CAD build for the part. Positions are in the model's coordinates, mm. A direction names the side the tool comes from. Round coordinates to 2 decimals unless told otherwise and drop trailing zeros. Order: outer loops, then holes, each group sorted by start corner. A loop starts at its lowest first (then second) coordinate and runs counter-clockwise, first axis right, second up. Notation, with made-up numbers: M -39,78 L -24,78 A30 cw -24,105 Z; hole C 23,-8.5 d9. An arc over 180 degrees is marked long. Answer as CSV lines item,"result". Start each with the question number.
```python
from build123d import *

# Parameters (mm, degrees)
BOSS_EXTRUDE2_DEPTH      = 25.4
CUT_EXTRUDE2_START       = 50.900485433
CUT_EXTRUDE2_OUTLINE_W   = 50.8
CUT_EXTRUDE2_OUTLINE_H   = 25.4
CUT_EXTRUDE2_OUTLINE_W_2 = 44.45
CUT_EXTRUDE2_OUTLINE_H_2 = 19.05
CUT_EXTRUDE2_DEPTH       = 80


# Read off the part's stored shape, not the designer's step: Cut-Extrude2
with BuildPart() as part:
    # Sketch2 → Boss-Extrude2 (new body)
    with BuildSketch(Plane.XY):
        with BuildLine():
            Line((-25.4, 130.900485433), (25.4, 130.900485433))
            Line((25.4, 130.900485433), (25.4, 30.900485433))
            ThreePointArc((25.4, 30.900485433), (0, -40), (-25.4, 30.900485433))
            Line((-25.4, 30.900485433), (-25.4, 130.900485433))
        make_face()
        Polygon((-16.541112452, 22.766888123), (-10.26013758, 21.772079433), (-4.496681536, 23.64473982), (0, 28.141421356), (4.496681536, 23.64473982), (10.26013758, 21.772079433), (16.541112452, 22.766888123), (17.535921141, 16.485913251), (21.09793287, 11.583224708), (26.764082159, 8.696177445), (23.877034895, 3.030028156), (23.877034895, -3.030028156), (26.764082159, -8.696177445), (21.09793287, -11.583224708), (17.535921141, -16.485913251), (16.541112452, -22.766888123), (10.26013758, -21.772079433), (4.496681536, -23.64473982), (0, -28.141421356), (-4.496681536, -23.64473982), (-10.26013758, -21.772079433), (-16.541112452, -22.766888123), (-17.535921141, -16.485913251), (-21.09793287, -11.583224708), (-26.764082159, -8.696177445), (-23.877034895, -3.030028156), (-23.877034895, 3.030028156), (-26.764082159, 8.696177445), (-21.09793287, 11.583224708), (-17.535921141, 16.485913251), align=None, mode=Mode.SUBTRACT)
    extrude(amount=BOSS_EXTRUDE2_DEPTH)

    # Cut-Extrude2 outline → Cut-Extrude2 (cut)
    with BuildSketch(Plane(origin=(0, 0, 0), x_dir=(1, 0, 0), z_dir=(0, 1, 0)).offset(CUT_EXTRUDE2_START)):
        with Locations((0, -12.7)):
            Rectangle(CUT_EXTRUDE2_OUTLINE_W, CUT_EXTRUDE2_OUTLINE_H)
        with Locations((0, -12.7)):
            Rectangle(CUT_EXTRUDE2_OUTLINE_W_2, CUT_EXTRUDE2_OUTLINE_H_2, mode=Mode.SUBTRACT)
    extrude(amount=CUT_EXTRUDE2_DEPTH, mode=Mode.SUBTRACT)


solid = part.part
```
Q1. Mould opens along X. For faces 4 (the cylindrical face through (1.374, -39.976, 12.522)), 5 (the flat face through (-2.22, -25.92, 12.52)), 6 (the flat face through (0, 90, 22.225)), 7 (the flat face through (-17.03, -19.67, 12.52)) say: +X half, -X half, draft (parallel to the pull), parting line (faces both ways), or undercut.
Q2. Band-saw the part on C-C, the plane y = 41.5. Write the cut outline in (x, z).
Q3. Band-saw the part on D-D, the plane x = -33.5. Write the cut outline in (y, z), then the cut area to 3 significant figures.
Q4. Drop flat-ended pins along their axis: P1, Ø1.8, axis at y = -1, z = 9.5, coming from the +X side; P2, Ø5, axis at x = 29, z = 21, coming from the -Y side; P3, Ø1.5, axis at y = 85.5, z = 10.5, coming from the +X side (3 decimals). Give the stop position or say it passes through.
Q5. Band-saw the part on B-B, the plane x = -8. Write the cut outline in (y, z) (3 decimals).
Q6. Band-saw the part on A-A, the plane y = 0. Write the cut outline in (x, z), then the cut area to 3 significant figures.
Q7. Probe line 1 along Z through (x, y) = (2.5, 77) (3 decimals); line 2 along X through (y, z) = (116, 9.25) (3 decimals); line 3 along Y through (x, z) = (20, 9). List the from-to ranges inside material, lowest first. Write a range as from..to.
Q8. Tool access for faces 1 (the flat face through (22.225, 90, 13)), 2 (the flat face through (0, 90, 3.175)), 3 (the flat face through (-25.34, -5.9, 12.52)): list every direction of +Z, -Z, +X, -X, +Y, -Y with a clear straight run to the whole face (end or side of a thin tool).
Answer:
1,face 4,"parting line"
1,face 5,"undercut"
1,face 6,"draft"
1,face 7,"undercut"
2,outline,"M -25.4,0 L 25.4,0 L 25.4,25.4 L -25.4,25.4 Z"
3,outline,"M -21.86,0 L 21.86,0 L 21.86,25.4 L -21.86,25.4 Z"
3,area,"1,110 mm^2"
4,P1,"stops at x = 40"
4,P2,"stops at y = -29.96"
4,P3,"stops at x = 22.225"
5,outline,"M -39.192,0 L -22.506,0 L -22.506,25.4 L -39.192,25.4 Z; M 22.506,0 L 50.9,0 L 50.9,3.175 L 130.9,3.175 L 130.9,22.225 L 50.9,22.225 L 50.9,25.4 L 22.506,25.4 Z"
6,outline,"M -40,0 L -23.88,0 L -23.88,25.4 L -40,25.4 Z; M 23.88,0 L 40,0 L 40,25.4 L 23.88,25.4 Z"
6,area,"819 mm^2"
7,line 1,"z = 3.175..22.225"
7,line 2,"x = -22.225..22.225"
7,line 3,"y = -34.64..-13.09, 13.09..130.9"
8,face 1,"+Z, -Z, +X, +Y"
8,face 2,"-Z, +X, -X, +Y"
8,face 3,"+Z, -Z"
